For this review, take the finished solid that the model builds, in its own axes (mm). A direction names the side the tool comes from. Round coordinates to 2 decimals unless told otherwise and drop trailing zeros. Order: outer loops, then holes, each group sorted by start corner. A loop starts at its lowest first (then second) coordinate and runs counter-clockwise, first axis right, second up. Notation, with made-up numbers: (-29.75, -39.75) -> (22.25, -39.75) arc R12 ccw to (22.25, -33.75) -> close; hole circle Ø9 at (-21.5, 69.5). An arc over 180 degrees is marked (long way). Answer in a Markdown table with one row per item.
```python
from build123d import *

# Parameters (mm, degrees)
ESQUISSE1_R        = 1.75
BOSS_EXTRU_1_DEPTH = 12
CHANFREIN1_SIZE    = 2


with BuildPart() as part:
    # Esquisse1 → Boss.-Extru.1 (new body)
    with BuildSketch(Plane(origin=(0, 0, 0), x_dir=(-1, 0, 0), z_dir=(0, 1, 0))):
        Polygon((-5.5, 3), (-2.5, 0), (2.5, 0), (5.5, 3), (2.5, 3), (2.5, 6), (4.5, 6), (4.5, 11), (-4.5, 11), (-4.5, 6), (-2.5, 6), (-2.5, 3), align=None)
        with Locations((0, 8.5)):
            Circle(ESQUISSE1_R, mode=Mode.SUBTRACT)
    extrude(amount=BOSS_EXTRU_1_DEPTH)

    # Chanfrein1
    chanfrein1_edges = [part.edges().sort_by_distance(p)[0] for p in [
        (4.5, 6, 11),
        (-4.5, 6, 11),
    ]]
    chamfer(chanfrein1_edges, length=CHANFREIN1_SIZE)


solid = part.part
```
Q1. Tool access review of faces 1 (the face through (4, 6, 6)), 2 (the face through (-4.5, 6, 7)), 3 (the face through (4.5, 6, 8)), 4 (the face through (-4, 6, 3)), 5 (the face through (-4, 5.9, 1.5)): name each direction out of +Z, -Z, +X, -X, +Y, -Y from which nothing blocks a thin tool from reaching the whole face with its end or side.
Answer key:
| item | result |
|---|---|
| face 1 | +X, +Y, -Y |
| face 2 | +Z, -X, +Y, -Y |
| face 3 | +Z, +X, +Y, -Y |
| face 4 | -X, +Y, -Y |
| face 5 | -Z, -X, +Y, -Y |
Q2. Clearance check with flat-ended pins moving along their axes: pin 1 Ø1 at (x, y) = (3.5, 5.5) entering from -Z; pin 2 Ø1.5 at (x, y) = (-3.5, 5.5) entering from +Z; pin 3 Ø0.9 at (y, z) = (7, 7) entering from +X. State where each tip first meets the part, or that it passes through.
Answer key:
| item | result |
|---|---|
| pin 1 | stops at z = 0.5 |
| pin 2 | stops at z = 10.75 |
| pin 3 | stops at x = 4.5 |
Q3. The part is to be moulded in two halves that separate along X. For faces 6 (the face through (-3.5, 5.9, 10)), 7 (the face through (-3, 6, 6)), 8 (the face through (0.228, 5.916, 10.235)), 9 (the face through (2.5, 6, 5)), say which applies: +X half, -X half, draft (parallel to the pull), parting line (faces both ways), or undercut.
Answer key:
| item | result |
|---|---|
| face 6 | -X half |
| face 7 | draft |
| face 8 | undercut |
| face 9 | +X half |
Q4. Take a section at B-B, the plane z = 8.5. Write out the cut boundary in (x, y), then the cut area to 3 significant figures.
Answer key:
| item | result |
|---|---|
| outline | (-4.5, 0) -> (-1.75, 0) -> (-1.75, 12) -> (-4.5, 12) -> close; (1.75, 0) -> (4.5, 0) -> (4.5, 12) -> (1.75, 12) -> close |
| area | 66.0 mm^2 |
Q5. Take a section at A-A, the plane x = 0. Write out the cut boundary in (y, z), then the cut area to 3 significant figures.
Answer key:
| item | result |
|---|---|
| outline | (0, 0) -> (12, 0) -> (12, 6.75) -> (0, 6.75) -> close; (0, 10.25) -> (12, 10.25) -> (12, 11) -> (0, 11) -> close |
| area | 90.0 mm^2 |
Q6. Take a section at D-D, the plane z = 2. Write out the cut boundary in (x, y).
Answer key:
| item | result |
|---|---|
| outline | (-4.5, 0) -> (4.5, 0) -> (4.5, 12) -> (-4.5, 12) -> close |
Q7. Take a section at C-C, the plane y = 6. Write out the cut boundary in (x, z), then the cut area to 3 significant figures.
Answer key:
| item | result |
|---|---|
| outline | (-5.5, 3) -> (-2.5, 0) -> (2.5, 0) -> (5.5, 3) -> (2.5, 3) -> (2.5, 6) -> (4.5, 6) -> (4.5, 9) -> (2.5, 11) -> (-2.5, 11) -> (-4.5, 9) -> (-4.5, 6) -> (-2.5, 6) -> (-2.5, 3) -> close; hole circle Ø3.5 at (0, 8.5) |
| area | 70.4 mm^2 |
Q8. To check wall thickness, follow probe 1 along Z at (x, y) = (0, 5.5); probe 2 along X at (y, z) = (0.5, 10); probe 3 along Z at (x, y) = (-5, 11). State the ranges of each line that lie inside material, in increasing order.
Answer key:
| item | result |
|---|---|
| probe 1 | z = 0 to 6.75, 10.25 to 11 |
| probe 2 | x = -3.5 to -0.9, 0.9 to 3.5 |
| probe 3 | z = 2.5 to 3 |
